Work out the finished part from the listing and answer in its coordinate system (mm). Face numbers are marked on the shaded views. A direction names the side the tool comes from. Coordinates: 2 decimals unless noted, no trailing zeros. Order: outer loops, then holes, each group sorted by start corner. A loop starts at its lowest first (then second) coordinate and runs counter-clockwise, first axis right, second up. Notation, with made-up numbers: M 49.25,77.5 L 104.25,77.5 A23 ccw 104.25,102.5 Z; hole C -2.75,48.25 d3. An arc over 180 degrees is marked long. Write item = value, one per line. Start each with the question number.
Q1. Straight lines are drawn through the part: line 1 along X through (y, z) = (-1, 0); line 2 along X through (y, z) = (8, -2.75); line 3 along Y through (x, z) = (3.5, -0.5). For each, find the intervals that lie inside material, in ascending order.
Q2. A tool of negligible diameter and unlimited length cuts with its end or side. For the marked faces 1, 2, 3 and 4, from which of +Z, -Z, +X, -X, +Y, -Y can it reach the whole face along a straight path? Write none if from no direction.
Q3. Each of these flat-tipped pins is pushed along its axis until it touches: P1, Ø4.5, axis at y = 3, z = 10, coming from the +X side; P2, Ø1, axis at x = 2, y = -7, coming from the +Z side; P3, Ø1, axis at x = -16, z = 5.5, coming from the -Y side; P4, Ø12, axis at x = 15, y = 8, coming from the -Z side. Where does it stop, or does it pass through?
Q4. Determine the mould class of the marked faces 5, 6 and 7 for opening direction X: released by +X, released by -X, zero draft, split by the parting line, or undercut.
Q5. Find section B-B on x = 2.5. Give the vertices of the cut face in (y, z).
Q6. Find section A-A on y = 0. Give the number of separate pieces and of enclosed holes in the cut face, and give its area (3 significant figures).
```python
from build123d import *

# Parameters (mm, degrees)
F1_DEPTH  = 12.5
F3_DEPTH  = 9
F4_W      = 10
F4_H      = 5
F6_R      = 3
F7_R      = 2
F8_DEPTH  = 5
F9_W      = 4
F9_H      = 20
F10_DEPTH = 12
F11_DEPTH = 0.7


with BuildPart() as f1:
    # F0 (on Front) → F1 (new body, symmetric)
    with BuildSketch(Plane.XZ):
        with BuildLine():
            Line((-35.5, 7.5), (-12.409673646, 7.5))
            ThreePointArc((-12.409673646, 7.5), (7.1239034244, -12.6293309403), (0, 14.5))
            Line((0, 14.5), (-35.5, 14.5))
            Line((-35.5, 14.5), (-35.5, 7.5))
        make_face()
    extrude(amount=F1_DEPTH, both=True)

    # F2 (on Front) → F3 (cut, symmetric)
    with BuildSketch(Plane.XZ):
        with BuildLine():
            Line((-10.5, 11.5), (-10.5, 5.8094750193))
            ThreePointArc((-10.5, 5.8094750193), (7.7746445838, -9.1408370292), (-4.0490846521, 11.2962344823))
            Line((-4.0490846521, 11.2962344823), (1.5, 14.5))
            Line((1.5, 14.5), (-10.5, 14.5))
            Line((-10.5, 14.5), (-10.5, 12.5))
            Line((-10.5, 12.5), (-35.5, 12.5))
            Line((-35.5, 12.5), (-35.5, 9))
            Line((-35.5, 9), (-10.5, 11.5))
        make_face()
    extrude(amount=F3_DEPTH, both=True, mode=Mode.SUBTRACT)

    # F4 (on Front) → F5 (revolve)
    with BuildSketch(Plane.XZ):
        with Locations((16.9203263894, 2.5)):
            Rectangle(F4_W, F4_H)
    revolve(axis=Axis((16.9203263894, 0, 0), (1, 0, 0)))

    # F6
    f6_edges = [f1.edges().sort_by_distance(p)[0] for p in [
        (21.920326, 0, -5),
    ]]
    fillet(f6_edges, radius=F6_R)

    # F7 (on Front) → F8 (cut, symmetric)
    with BuildSketch(Plane.XZ):
        with Locations((16.9203263894, 0)):
            Circle(F7_R)
    extrude(amount=F8_DEPTH, both=True, mode=Mode.SUBTRACT)

    # F9 (on face) → F10 (join)
    with BuildSketch(Plane(origin=(0, 0, 7.5), x_dir=(1, 0, 0), z_dir=(0, 0, -1))):
        with Locations((-33.5, 0)):
            Rectangle(F9_W, F9_H)
    extrude(amount=F10_DEPTH)

    # F9 (on face) → F11 (join)
    with BuildSketch(Plane(origin=(0, 0, 7.5), x_dir=(1, 0, 0), z_dir=(0, 0, -1))):
        with Locations((-33.5, 0)):
            Rectangle(F9_W, F9_H)
    extrude(amount=F11_DEPTH)


solid = f1.part
```
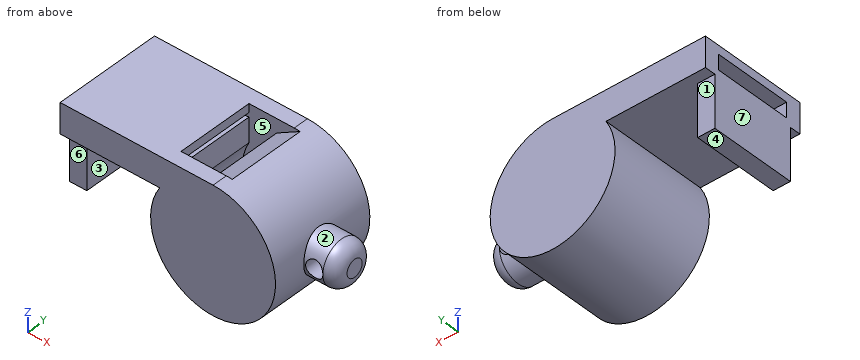
Findings below:
q1.line_1 = -35.5 to -31.5, -14.5 to -12, 11.92 to 14.92, 18.92 to 21.92
q1.line_2 = -35.5 to -31.5, -14.24 to -11.68, 11.68 to 14.24
q1.line_3 = -12.5 to -9, 9 to 12.5
q2.face_1 = -Z, -X, +Y
q2.face_2 = +X
q2.face_3 = -Z, +Y, -Y
q2.face_4 = -Z, -X, +Y, -Y
q3.P1 = 12.26
q3.P2 = 14.42
q3.P3 = through
q3.P4 = -11.37
q4.face_5 = undercut
q4.face_6 = zero draft
q4.face_7 = released by -X
q5.outline = M -12.5,-14.28 L 12.5,-14.28 L 12.5,14.28 L -12.5,14.28 Z; hole M -9,-11.74 L 9,-11.74 L 9,11.74 L -9,11.74 Z
q6.separate_pieces = 2
q6.enclosed_holes = 1
q6.area = 405 mm^2
